Can you work these out from the drawing? Everything is in mm from the part's minimum corner. Give positions to 0.01 mm unless a question says otherwise; leave off trailing zeros. Order: outer loops, then holes, each group sorted by start corner. A loop starts at its lowest first (then second) coordinate and runs counter-clockwise, first axis right, second up. Notation, with made-up numbers: (77, 26) - (96, 26) arc R19 ccw to (96, 48) - close; hole circle Ø8 at (37, -8.75). An arc over 180 degrees is marked (long way). Answer as a JSON object with one key per item and string values.
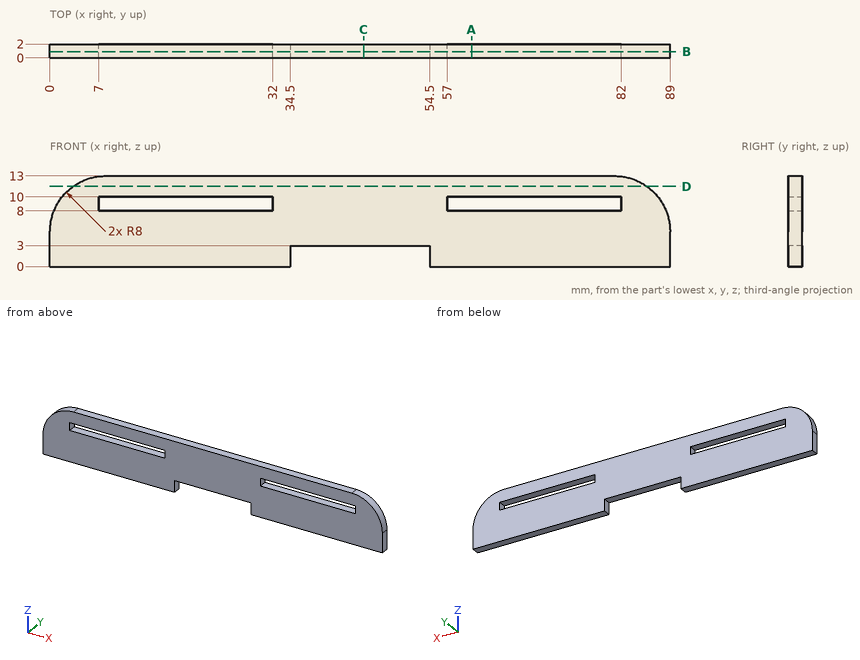
Q1. If we section it at A-A, the plane x = 60.5: Please give me the cut outline in (y, z), then the cut area to 3 significant figures.
Recorded:
{"outline": "(0, 0) - (2, 0) - (2, 8) - (0, 8) - close; (0, 10) - (2, 10) - (2, 13) - (0, 13) - close", "area": "22.0 mm^2"}
Q2. I need wall thicknesses on L1, parallel to Z at x = 75, y = 0.75; L2, parallel to X at y = 1.4, z = 9.5; L3, parallel to X at y = 1.55, z = 1.5. Which ranges of each line are inside material? Lowest first, please.
Recorded:
{"L1": "z = 0 to 8, 10 to 13", "L2": "x = 1.39 to 7, 32 to 57, 82 to 87.61", "L3": "x = 0 to 34.5, 54.5 to 89"}
Q3. If we section it at B-B, the plane y = 0.9: Please give me the cut outline in (x, z).
Recorded:
{"outline": "(0, 0) - (34.5, 0) - (34.5, 3) - (54.5, 3) - (54.5, 0) - (89, 0) - (89, 5) arc R8 ccw to (81, 13) - (8, 13) arc R8 ccw to (0, 5) - close; hole (7, 8) - (32, 8) - (32, 10) - (7, 10) - close; hole (57, 8) - (82, 8) - (82, 10) - (57, 10) - close"}
Q4. If we section it at D-D, the plane z = 11.5: Please give me the cut outline in (x, y), then the cut area to 3 significant figures.
Recorded:
{"outline": "(3.34, 0) - (85.66, 0) - (85.66, 2) - (3.34, 2) - close", "area": "165 mm^2"}
Q5. If we section it at C-C, the plane x = 45: Please give me the cut outline in (y, z), then the cut area to 3 significant figures.
Recorded:
{"outline": "(0, 3) - (2, 3) - (2, 13) - (0, 13) - close", "area": "20.0 mm^2"}
Q6. I'm going to push flat-ended pins straight in: pin 1 Ø0.6 at (y, z) = (0.5, 8.5) entering from -X; pin 2 Ø1 at (y, z) = (1.5, 9) entering from +X; pin 3 Ø0.6 at (y, z) = (1.5, 8.5) entering from +X. Where does each tip first touch, or does it pass through?
Recorded:
{"pin 1": "stops at x = 0.67", "pin 2": "stops at x = 88.19", "pin 3": "stops at x = 88.33"}
